from build123d import *

# Parameters (mm, degrees)
F1_DEPTH = 30
F2_R     = 1
F3_R     = 0.9999
F4_R     = 0.99999


# Not quite as in the source:
# - a fillet or chamfer is up to 0.001 mm smaller than in the source, because OpenCascade refuses the exact size


with BuildPart() as f1:
    # F0 (on Right) → F1 (new body)
    with BuildSketch(Plane.YZ):
        with BuildLine():
            Line((0, 8), (-1, 8))
            Line((-1, 8), (-2, 8))
            ThreePointArc((-2, 8), (-4.4792027106, 2.4792027106), (-10, 0))
            Line((-10, 0), (-11, 0))
            ThreePointArc((-11, 0), (-16.5207972894, 2.4792027106), (-19, 8))
            Line((-19, 8), (-20.9965492395, 8))
            Line((-20.9965492395, 8), (-20.9965492395, 7.8825559271))
            ThreePointArc((-20.9965492395, 7.8825559271), (-17.9350112011, 1.0649887989), (-11.1174440729, -1.9965492395))
            Line((-11.1174440729, -1.9965492395), (-9.8825559561, -1.9965487463))
            ThreePointArc((-9.8825559561, -1.9965487463), (-4.6211597315, -0.2176837422), (-1, 3.9934744279))
            ThreePointArc((-1, 3.9934744279), (2.6211597315, -0.2176837422), (7.8825559561, -1.9965487463))
            Line((7.8825559561, -1.9965487463), (9.1174440439, -1.9965487463))
            ThreePointArc((9.1174440439, -1.9965487463), (15.9350108518, 1.0649891482), (18.9965487463, 7.8825559561))
            Line((18.9965487463, 7.8825559561), (18.9965487463, 8))
            Line((18.9965487463, 8), (17, 8))
            ThreePointArc((17, 8), (14.5207972894, 2.4792027106), (9, 0))
            Line((9, 0), (8, 0))
            ThreePointArc((8, 0), (2.4792027106, 2.4792027106), (0, 8))
        make_face()
    extrude(amount=F1_DEPTH)

    # F2
    f2_edges = [f1.edges().sort_by_distance(p)[0] for p in [
        (15, -19, 8),
    ]]
    fillet(f2_edges, radius=F2_R)

    # F3 (radius 1 in the source; OpenCascade refuses exactly that, so slightly less here)
    f3_edges = [f1.edges().sort_by_distance(p)[0] for p in [
        (15, -20.996549, 8),
    ]]
    fillet(f3_edges, radius=F3_R)

    # F4 (radius 1 in the source; OpenCascade refuses exactly that, so slightly less here)
    f4_edges = [f1.edges().sort_by_distance(p)[0] for p in [
        (15, -2, 8),
        (15, 0, 8),
        (15, 18.996549, 8),
        (15, 17, 8),
    ]]
    fillet(f4_edges, radius=F4_R)


solid = f1.part
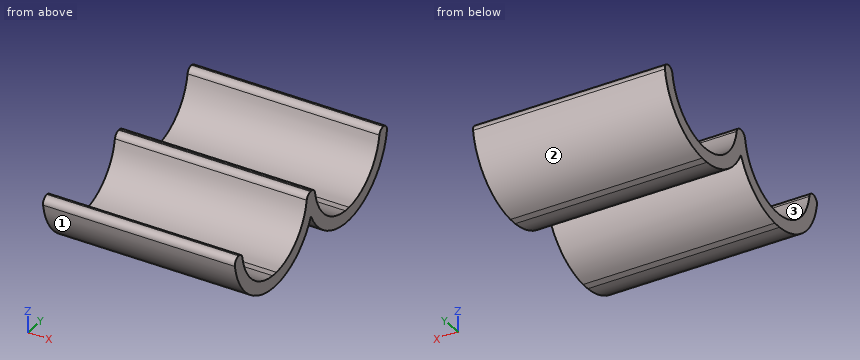
Work out the finished part from the listing and answer in its coordinate system (mm). Face numbers are marked on the shaded views. Round coordinates to 2 decimals unless told otherwise and drop trailing zeros. Write each loop counter-clockwise with the first axis right and the second up, starting at its lowest first coordinate (ties: lowest second). Pieces come first, ordered by that corner, then holes.
1) The mould has two halves that part along Y. Classify the marked faces 1, 2 and 3: pulls with the +Y half, pulls with the -Y half, needs draft (parallel to the pull), parting line crosses it, or undercut.
2) A cutting plane is placed at D-D (z = 0.75). Give the vertices of the cut face in (x, y).
3) Straight lines are drawn through the part: line 1 (Y direction, x = 21, z = 1.25); line 2 (Y direction, x = 7.5, z = 4.5); line 3 (Y direction, x = 23, z = 3.25). For each, find the intervals that lie inside material, in ascending order.
4) A cutting plane is placed at B-B (z = 2.75). Give the vertices of the cut face in (x, y).
5) Given pin 1 Ø5 at (x, y) = (14.5, 4) entering from -Z; pin 2 Ø5 at (x, z) = (3.5, 2.5) entering from -Y; pin 3 Ø2 at (x, y) = (23.5, -3) entering from -Z, each flat-ended and moving along its own axis, determine where each tip first touches the part or whether it passes through.
6) A cutting plane is placed at C-C (y = 7). Give the vertices of the cut face in (x, z).
7) A cutting plane is placed at A-A (z = -1.25). Give the vertices of the cut face in (x, y).
Completed:
1. face 1: pulls with the -Y half
1. face 2: pulls with the +Y half
1. face 3: undercut
2. outline: (0, -17.61) - (30, -17.61) - (30, -14.03) - (0, -14.03) - close; (0, -6.97) - (30, -6.97) - (30, -3.39) - (0, -3.39) - close; (0, 1.39) - (30, 1.39) - (30, 4.97) - (0, 4.97) - close; (0, 12.03) - (30, 12.03) - (30, 15.61) - (0, 15.61) - close
3. line 1: y = -18.12 to -14.97, -6.03 to -2.88, 0.88 to 4.03, 12.97 to 16.12
3. line 2: y = -20.22 to -18.02, -2.98 to 0.98, 16.02 to 18.22
3. line 3: y = -19.61 to -17.2, -3.8 to -1.39, -0.61 to 1.8, 15.2 to 17.61
4. outline: (0, -19.3) - (30, -19.3) - (30, -16.78) - (0, -16.78) - close; (0, -4.22) - (30, -4.22) - (30, -1.7) - (0, -1.7) - close; (0, -0.3) - (30, -0.3) - (30, 2.22) - (0, 2.22) - close; (0, 14.78) - (30, 14.78) - (30, 17.3) - (0, 17.3) - close
5. pin 1: stops at z = -1.82
5. pin 2: stops at y = -20.42
5. pin 3: stops at z = 0.24
6. outline: (0, -1.91) - (30, -1.91) - (30, 0.12) - (0, 0.12) - close
7. outline: (0, -14.44) - (30, -14.44) - (30, -6.56) - (0, -6.56) - close; (0, 4.56) - (30, 4.56) - (30, 12.44) - (0, 12.44) - close
